```python
from build123d import *

# Parameters (mm, degrees)
SKETCH001_W            = 182
SKETCH001_H            = 190
PAD_DEPTH              = 4
SKETCH154_R            = 1.85
POCKET004_DEPTH        = 130.001
LINEARPATTERN005_COUNT = 3
LINEARPATTERN005_PITCH = 91


with BuildPart() as part:
    # Sketch001 → Pad (new body)
    with BuildSketch(Plane.XY):
        with Locations((0, -5)):
            Rectangle(SKETCH001_W, SKETCH001_H)
        Polygon((-65, 76), (0, 6), (65, 76), align=None, mode=Mode.SUBTRACT)
        Polygon((-71, 70), (-6, 0), (-71, -70), align=None, mode=Mode.SUBTRACT)
        Polygon((-65, -76), (0, -6), (65, -76), align=None, mode=Mode.SUBTRACT)
        Polygon((71, -70), (6, 0), (71, 70), align=None, mode=Mode.SUBTRACT)
    extrude(amount=PAD_DEPTH)

    # Sketch154 → Pocket004 (cut, through all)
    with BuildSketch(Plane.XY.offset(130)):
        with Locations((-85, 86)):
            Circle(SKETCH154_R)
        with Locations((85, 86)):
            Circle(SKETCH154_R)
    pocket004 = extrude(amount=-POCKET004_DEPTH, mode=Mode.SUBTRACT)

    # LinearPattern005: Pocket004 ×3
    with Locations(*[(0, -i * LINEARPATTERN005_PITCH, 0) for i in range(1, LINEARPATTERN005_COUNT)]):
        add(pocket004, mode=Mode.SUBTRACT)


with BuildPart() as part_1:
    # Body placement: moved
    add(part.part.moved(Location((0, 0, 4))))


solid = part_1.part
```
Work out the finished part from the listing and answer in its coordinate system (mm). A direction names the side the tool comes from. Coordinates: 2 decimals unless noted, no trailing zeros. Write each loop counter-clockwise with the first axis right and the second up, starting at its lowest first coordinate (ties: lowest second). Pieces come first, ordered by that corner, then holes. Notation, with made-up numbers: (42.25, -19) - (82.25, -19) arc R23 ccw to (82.25, -7) - close; hole circle Ø11 at (-13, 33). An arc over 180 degrees is marked (long way). Answer as a JSON object with one key per item and string values.
Q1. For a pull along X with two mould halves and no side action, classify faces 1 (the flat face through (38.045, 34.51, 5.972)), 2 (the flat face through (-1, -4, 8)), 3 (the flat face through (-91, -6, 6)), 4 (the flat face through (91, -6, 6)) as pulls with the +X half, pulls with the -X half, needs draft (parallel to the pull), parting line crosses it, or undercut.
Results list:
{"face 1": "undercut", "face 2": "needs draft", "face 3": "pulls with the -X half", "face 4": "pulls with the +X half"}
Q2. Find section B-B (x = 19). Write down the section's boundary in (y, z).
Results list:
{"outline": "(-100, 4) - (-76, 4) - (-76, 8) - (-100, 8) - close; (-26.46, 4) - (-14, 4) - (-14, 8) - (-26.46, 8) - close; (14, 4) - (26.46, 4) - (26.46, 8) - (14, 8) - close; (76, 4) - (90, 4) - (90, 8) - (76, 8) - close"}
Q3. Which of the six approach directions +Z, -Z, +X, -X, +Y, -Y give full straight-line access (tool end or side, diameter ignored) to faces 5 (the flat face through (1, -76, 6)), 6 (the flat face through (-1, 90, 6))?
Results list:
{"face 5": "+Z, -Z", "face 6": "+Z, -Z, +X, -X, +Y"}
Q4. Find section C-C (x = -67.5). Write down the section's boundary in (y, z).
Results list:
{"outline": "(-100, 4) - (-66.23, 4) - (-66.23, 8) - (-100, 8) - close; (66.23, 4) - (90, 4) - (90, 8) - (66.23, 8) - close"}
Q5. Given pin 1 Ø3.5 at (x, y) = (85, -96) entering from -Z; pin 2 Ø5 at (x, y) = (85, -5) entering from -Z, each flat-ended and moving along its own axis, determine where each tip first touches the part or whether it passes through.
Results list:
{"pin 1": "passes through", "pin 2": "stops at z = 4"}
Q6. Consider L1, parallel to Y at x = -85, z = 6.4; L2, parallel to X at y = 86, z = 5.55; L3, parallel to Y at x = -18, z = 4.9. Determine where each line is inside the solid, lowest interval first. Write a range as from..to.
Results list:
{"L1": "y = -100..-97.85, -94.15..-6.85, -3.15..84.15, 87.85..90", "L2": "x = -91..-86.85, -83.15..83.15, 86.85..91", "L3": "y = -100..-76, -25.38..-12.92, 12.92..25.38, 76..90"}
Q7. Find section A-A (z = 5.1). State how many separate pieces and enclosed holes the cut face has, plus the area to 3 significant figures.
Results list:
{"separate pieces": "1", "enclosed holes": "10", "area": "16,300 mm^2"}
Q8. Find section D-D (y = -53.5). Write down the section's boundary in (x, z).
Results list:
{"outline": "(-91, 4) - (-71, 4) - (-71, 8) - (-91, 8) - close; (-55.68, 4) - (-44.11, 4) - (-44.11, 8) - (-55.68, 8) - close; (44.11, 4) - (55.68, 4) - (55.68, 8) - (44.11, 8) - close; (71, 4) - (91, 4) - (91, 8) - (71, 8) - close"}
